```python
from build123d import *

# Parameters (mm, degrees)
F0_R     = 0.8
F1_DEPTH = 8
F0_R_2   = 1.9
F2_DEPTH = 0.5
F4_DEPTH = 0.4


with BuildPart() as f1:
    # F0 (on Top) → F1 (new body)
    with BuildSketch(Plane.XY):
        Circle(F0_R)
    extrude(amount=F1_DEPTH)

    # F0 (on Top) → F2 (join)
    with BuildSketch(Plane.XY):
        Circle(F0_R_2)
        Circle(F0_R, mode=Mode.SUBTRACT)
    extrude(amount=F2_DEPTH)

    # F3 (on face) → F4 (cut)
    with BuildSketch(Plane(origin=(0, 0, 0), x_dir=(1, 0, 0), z_dir=(0, 0, -1))):
        Polygon((0.521101, -0.900798), (1.040665, 0.000888), (0.519563, 0.901686), (-0.521101, 0.900798), (-1.040665, -0.000888), (-0.519563, -0.901686), align=None)
    extrude(amount=-F4_DEPTH, mode=Mode.SUBTRACT)


solid = f1.part
```
The listing builds one solid part. Answer for the finished solid, in the listing's coordinates (mm). A direction names the side the tool comes from. Give positions to 0.01 mm unless a question says otherwise; leave off trailing zeros. Write each loop counter-clockwise with the first axis right and the second up, starting at its lowest first coordinate (ties: lowest second). Pieces come first, ordered by that corner, then holes. Notation, with made-up numbers: (31.5, 88) -> (41.5, 88) arc R21 cw to (41.5, 94) -> close; hole circle Ø3 at (-25, -5). An arc over 180 degrees is marked (long way). Write item = value, one per line. Start each with the question number.
1) Straight lines are drawn through the part: line 1 along Z through (x, y) = (0.7, 1.5); line 2 along Y through (x, z) = (0.6, 1.75); line 3 along Y through (x, z) = (-0.7, 3). For each, find the intervals that lie inside material, in ascending order.
2) The part is cut by section C-C, the plane y = 0.55. Determine the outline of the cut face in (x, z), and give its area (3 significant figures).
3) The part is cut by section A-A, the plane x = 0.4. Determine the outline of the cut face in (y, z).
4) The part is cut by section D-D, the plane x = 1.55. Determine the outline of the cut face in (y, z).
5) Which of the six approach directions +Z, -Z, +X, -X, +Y, -Y give full straight-line access (tool end or side, diameter ignored) to faces 1 (the face through (-0.63, -0.49, 4.2)), 2 (the face through (0, 0, 8))?
6) The part is cut by section B-B, the plane z = 6.25. Determine the outline of the cut face in (x, y), and give its area (3 significant figures).
7) This flat-tipped pin is pushed along its axis until it touches: pin 1 (1.1 mm diameter, centred on x = 0, y = -1, fed in from +Z). Where does it stop, or does it pass through?
8) Determine the mould class of faces 3 (the face through (-1.9, 0.08, 0.25)), 4 (the face through (0, 0, 0.4)), 5 (the face through (1, -1, 0)) for opening direction Y: +Y half, -Y half, draft (parallel to the pull), parting line (faces both ways), or undercut.
Solutions:
q1.line_1 = 0 to 0.5
q1.line_2 = -0.53 to 0.53
q1.line_3 = -0.39 to 0.39
q2.outline = (-1.82, 0) -> (-0.72, 0) -> (-0.72, 0.4) -> (0.72, 0.4) -> (0.72, 0) -> (1.82, 0) -> (1.82, 0.5) -> (0.58, 0.5) -> (0.58, 8) -> (-0.58, 8) -> (-0.58, 0.5) -> (-1.82, 0.5) -> close
q2.area = 9.95 mm²
q3.outline = (-1.86, 0) -> (-0.9, 0) -> (-0.9, 0.4) -> (0.9, 0.4) -> (0.9, 0) -> (1.86, 0) -> (1.86, 0.5) -> (0.69, 0.5) -> (0.69, 8) -> (-0.69, 8) -> (-0.69, 0.5) -> (-1.86, 0.5) -> close
q4.outline = (-1.1, 0) -> (1.1, 0) -> (1.1, 0.5) -> (-1.1, 0.5) -> close
q5.face_1 = +Z
q5.face_2 = +Z, +X, -X, +Y, -Y
q6.outline = circle Ø1.6 at (0, 0)
q6.area = 2.01 mm²
q7.pin_1 = 8
q8.face_3 = parting line
q8.face_4 = undercut
q8.face_5 = draft
